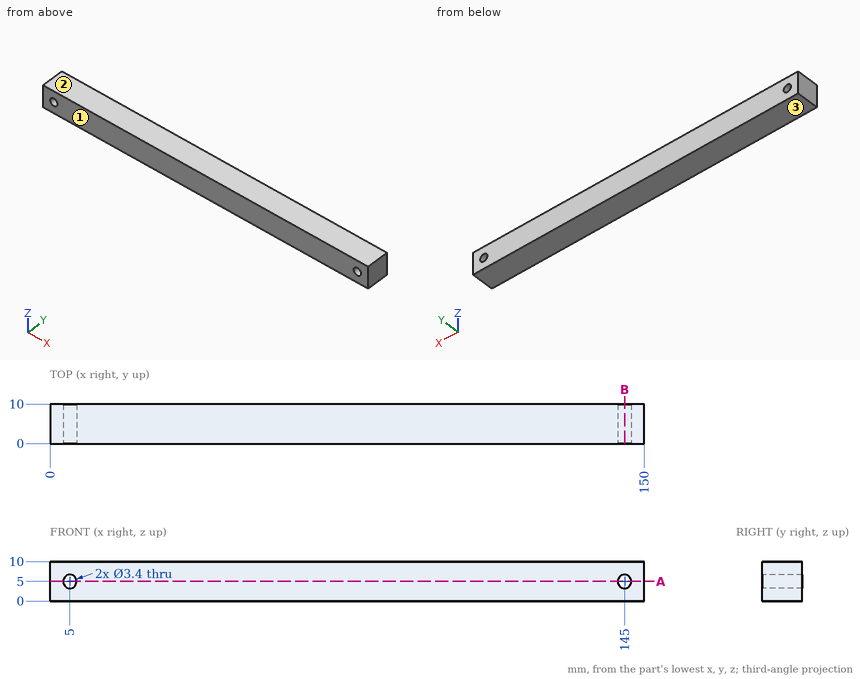
For this review, use the dimensioned drawing (mm, ordinates from the lowest corner) and the shaded views. Coordinates: 2 decimals unless noted, no trailing zeros. Order: outer loops, then holes, each group sorted by start corner. A loop starts at its lowest first (then second) coordinate and runs counter-clockwise, first axis right, second up. Notation, with made-up numbers: M 38,22.5 L 45,22.5 A18 ccw 45,28.5 Z; hole C -6.5,-36.75 d7. An arc over 180 degrees is marked long. Answer as a JSON object with one key per item and string values. Group by question number.
1) Mouldability with a two-part tool opening along Z and no side actions: class the marked faces 1, 2 and 3 as pulls with the +Z half, pulls with the -Z half, needs draft (parallel to the pull), parting line crosses it, or undercut.
2) Add section A-A, the plane z = 5. Write out the cut boundary in (x, y).
3) For pin 1 (2 mm diameter, centred on x = 145, z = 5, fed in from +Y), flat-tipped, find the tip position at first contact; note if it passes through.
4) Add section B-B, the plane x = 145. Write out the cut boundary in (y, z).
5) Wall thickness on L1, parallel to X at y = 1, z = 5.25; L2, parallel to Z at x = 5, y = 3.5; L3, parallel to X at y = 7.75, z = 4.5: over which ranges is each line inside the solid? List them lowest first.
Computed values:
{
 "1": {"face 1": "needs draft", "face 2": "pulls with the +Z half", "face 3": "pulls with the -Z half"},
 "2": {"outline": "M 0,0 L 3.3,0 L 3.3,10 L 0,10 Z; M 6.7,0 L 143.3,0 L 143.3,10 L 6.7,10 Z; M 146.7,0 L 150,0 L 150,10 L 146.7,10 Z"},
 "3": {"pin 1": "passes through"},
 "4": {"outline": "M 0,0 L 10,0 L 10,3.3 L 0,3.3 Z; M 0,6.7 L 10,6.7 L 10,10 L 0,10 Z"},
 "5": {"L1": "x = 0 to 3.32, 6.68 to 143.32, 146.68 to 150", "L2": "z = 0 to 3.3, 6.7 to 10", "L3": "x = 0 to 3.38, 6.62 to 143.38, 146.62 to 150"}
}
